Autodesk Inventor part; units mm, degrees
ref_plane "YZ Plane" through (0, 0, 0) normal (1, 0, 0) x (0, 1, 0)
ref_plane "XZ Plane" through (0, 0, 0) normal (0, 1, 0) x (-1, 0, 0)
ref_plane "XY Plane" through (0, 0, 0) normal (0, 0, 1) x (1, 0, 0)
ref_plane "Work Plane1" through (0, 0, 0) normal (0, 0, 1) x (1, 0, 0)
sketch "Sketch1" plane through (0, 0, 0) normal (0, 0, 1) x (1, 0, 0)
  line L0 (498, -287.5204) -> (0, -575.0409)
  line L1 (0, -575.0409) -> (-498, -287.5204)
  line L2 (-498, -287.5204) -> (-498, 287.5204)
  line L3 (-498, 287.5204) -> (0, 575.0409)
  line L4 (0, 575.0409) -> (498, 287.5204)
  line L5 (498, 287.5204) -> (498, -287.5204)
  line L6 (300, -173.2051) -> (0, -346.4102)
  line L7 (0, -346.4102) -> (-300, -173.2051)
  line L8 (-300, -173.2051) -> (-300, 173.2051)
  line L9 (-300, 173.2051) -> (0, 346.4102)
  line L10 (0, 346.4102) -> (300, 173.2051)
  line L11 (300, 173.2051) -> (300, -173.2051)
  point P0 (0, 0)
  point P1 (0, 0)
  point P2 (0, 0)
  dimension "d0" = 300
  dimension "d1" = 498
extrude "Extrusion1" add sketch "Sketch1" along normal blind 50
properties part number "Electrical" material "Acetal Resin, White"
Geometry check sheet. Reference: the model listing, model coordinates, mm. A direction names the side the tool comes from. Coordinates: 2 decimals unless noted, no trailing zeros. Order: outer loops, then holes, each group sorted by start corner. A loop starts at its lowest first (then second) coordinate and runs counter-clockwise, first axis right, second up. Notation, with made-up numbers: (14.25, 28) - (53.25, 28) arc R15 cw to (53.25, 34) - close; hole circle Ø8 at (67.25, 64). An arc over 180 degrees is marked (long way). Answer in a Markdown table with one row per item. Add a question column.
1) Gauge pin test, flat ends, axial feed: P1, Ø2, axis at x = 317, z = 44, coming from the -Y side; P2, Ø6, axis at x = 91, z = 28, coming from the -Y side; P3, Ø4, axis at x = -248, z = 25.5, coming from the +Y side; P4, Ø1.5, axis at x = -77, y = 343.5, coming from the -Z side. Record the tip position at first contact, or that the pin passes through.
2) Cross-section at A-A, the plane y = 77. Record the cut outline in (x, z), then the cut area to 3 significant figures.
3) Cross-section at C-C, the plane x = 110.5. Record the cut outline in (y, z), then the cut area to 3 significant figures.
4) Cross-section at D-D, the plane y = 488. Record the cut outline in (x, z), then the cut area to 3 significant figures.
5) Material ranges on line 1 along X through (y, z) = (133.5, 8); line 2 along X through (y, z) = (195, 19); line 3 along Y through (x, z) = (-77, 20.5), recorded low to high. Write a range as [from, to].
6) Release check for a two-part mould opening along Y. For faces 1 (the flat face through (-147.9, -261.02, 24.65)), 2 (the flat face through (245.5, 433.3, 24.6)), 3 (the flat face through (214, -248, 50)) record: +Y half, -Y half, draft (parallel to the pull), parting line (faces both ways), or undercut.
7) Cross-section at B-B, the plane z = 12. Record the cut outline in (x, y).
8) Set-up check for faces 4 (the flat face through (300, 2, 25)), 5 (the flat face through (-245.5, -433.3, 24.6)): record each of +Z, -Z, +X, -X, +Y, -Y from which the full face is reachable in a straight line by a thin tool's end or side.
Check result:
| question | item | result |
|---|---|---|
| 1 | P1 | stops at y = -392.6 |
| 1 | P2 | stops at y = -524.23 |
| 1 | P3 | stops at y = 433.01 |
| 1 | P4 | stops at z = 0 |
| 2 | outline | (-498, 0) - (-300, 0) - (-300, 50) - (-498, 50) - close; (300, 0) - (498, 0) - (498, 50) - (300, 50) - close |
| 2 | area | 19,800 mm² |
| 3 | outline | (-511.24, 0) - (-282.61, 0) - (-282.61, 50) - (-511.24, 50) - close; (282.61, 0) - (511.24, 0) - (511.24, 50) - (282.61, 50) - close |
| 3 | area | 22,900 mm² |
| 4 | outline | (-150.76, 0) - (150.76, 0) - (150.76, 50) - (-150.76, 50) - close |
| 4 | area | 15,100 mm² |
| 5 | line 1 | x = [-498, -300], [300, 498] |
| 5 | line 2 | x = [-498, -262.25], [262.25, 498] |
| 5 | line 3 | y = [-530.58, -301.95], [301.95, 530.58] |
| 6 | face 1 | undercut |
| 6 | face 2 | +Y half |
| 6 | face 3 | draft |
| 7 | outline | (-498, -287.52) - (0, -575.04) - (498, -287.52) - (498, 287.52) - (0, 575.04) - (-498, 287.52) - close; hole (-300, -173.21) - (0, -346.41) - (300, -173.21) - (300, 173.21) - (0, 346.41) - (-300, 173.21) - close |
| 8 | face 4 | +Z, -Z |
| 8 | face 5 | +Z, -Z, -X, -Y |
